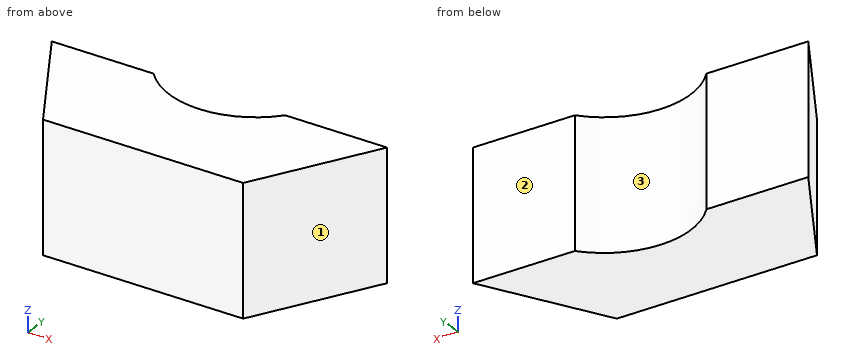
from build123d import *

# Parameters (mm, degrees)
SKETCH_1_R          = 20
EXTRUDE_1_DEPTH     = 30
SKETCH_2_W          = 102.73425285
SKETCH_2_H          = 41.168069265
CUT_EXTRUDE_1_DEPTH = 89
SKETCH_3_W          = 92.921845771
SKETCH_3_H          = 3
CUT_EXTRUDE_2_DEPTH = 89
SKETCH_5_W          = 89.254796613
SKETCH_5_H          = 10
CUT_EXTRUDE_3_DEPTH = 31


with BuildPart() as part:
    # 스케치1 → 보스-돌출1 (new body)
    with BuildSketch(Plane.XY):
        Polygon((46.188021535, 0), (23.094010768, 40), (-23.094010768, 40), (-46.188021535, 0), (-23.094010768, -40), (23.094010768, -40), align=None)
        Circle(SKETCH_1_R, mode=Mode.SUBTRACT)
    extrude(amount=EXTRUDE_1_DEPTH)

    # 스케치2 → 컷-돌출1 (cut)
    with BuildSketch(Plane.XY):
        with Locations((0.690561162, 20.584034632)):
            Rectangle(SKETCH_2_W, SKETCH_2_H)
    extrude(amount=CUT_EXTRUDE_1_DEPTH, mode=Mode.SUBTRACT)

    # 스케치3 → 컷-돌출2 (cut)
    with BuildSketch(Plane.XY.offset(30)):
        with Locations((-0.27290135, -1.5)):
            Rectangle(SKETCH_3_W, SKETCH_3_H)
    extrude(amount=-CUT_EXTRUDE_2_DEPTH, mode=Mode.SUBTRACT)

    # 스케치5 → 컷-돌출3 (cut, through all)
    with BuildSketch(Plane.XY.offset(30)):
        with Locations((-0.171427578, -8)):
            Rectangle(SKETCH_5_W, SKETCH_5_H)
    extrude(amount=-CUT_EXTRUDE_3_DEPTH, mode=Mode.SUBTRACT)


solid = part.part
Design review of the part built by this model. Coordinates are the model's own, in mm. Face numbers are marked on the shaded views. Give positions to 0.01 mm unless a question says otherwise; leave off trailing zeros. Loops run counter-clockwise (first coordinate to the right, second up) from the corner with the lowest first, then second, coordinate; pieces in that order, holes last. Notation, with made-up numbers: M 81,-31.5 L 140,-31.5 A7 cw 140,-18.5 Z; hole C 24.5,29.5 d3. An arc over 180 degrees is marked long. One line per question, with ' | ' between items. Start each with the question number.
1. Add section C-C (x = -10). Write out the cut boundary in (y, z), plus the area to 3 significant figures.
2. Add section A-A (y = -15.5). Write out the cut boundary in (x, z), plus the area to 3 significant figures.
3. To check wall thickness, follow L1, parallel to X at y = -16.75, z = 18.5; L2, parallel to X at y = -15.5, z = 18.25; L3, parallel to X at y = -37.5, z = 22.25. State the ranges of each line that lie inside material, in increasing order.
4. Add section D-D (y = -24.75). Write out the cut boundary in (x, z), plus the area to 3 significant figures.
5. Add section B-B (z = 19). Write out the cut boundary in (x, y), plus the area to 3 significant figures.
6. Insertion check: P1, Ø2, axis at y = -28, z = 23, coming from the +X side; P2, Ø4, axis at y = -27, z = 5.5, coming from the +X side; P3, Ø10, axis at y = -35.5, z = 21, coming from the +X side; P4, Ø10, axis at x = -10, y = -20.5, coming from the -Z side. Each pin has a flat end and moves straight along its axis. Give the tip position at first contact, or say it passes through.
7. The part is to be moulded in two halves that separate along X. For the marked faces 1, 2 and 3, say which applies: released by +X, released by -X, zero draft, split by the parting line, or undercut.
Worked out:
1) outline: M -40,0 L -17.32,0 L -17.32,30 L -40,30 Z | area: 680 mm²
2) outline: M -37.24,0 L -12.64,0 L -12.64,30 L -37.24,30 Z; M 12.64,0 L 37.24,0 L 37.24,30 L 12.64,30 Z | area: 1,480 mm²
3) L1: x = -36.52 to -10.93, 10.93 to 36.52 | L2: x = -37.24 to -12.64, 12.64 to 37.24 | L3: x = -24.54 to 24.54
4) outline: M -31.9,0 L 31.9,0 L 31.9,30 L -31.9,30 Z | area: 1,910 mm²
5) outline: M -38.68,-13 L -23.09,-40 L 23.09,-40 L 38.68,-13 L 15.2,-13 A20 cw -15.2,-13 Z | area: 1,520 mm²
6) P1: stops at x = 30.6 | P2: stops at x = 31.75 | P3: stops at x = 28.58 | P4: stops at z = 0
7) face 1: released by +X | face 2: zero draft | face 3: undercut
